Part print with two shaded views. Sizes in mm from the minimum x, y, z corner. A direction names the side the tool comes from. Give positions to 0.01 mm unless a question says otherwise; leave off trailing zeros. Order: outer loops, then holes, each group sorted by start corner. A loop starts at its lowest first (then second) coordinate and runs counter-clockwise, first axis right, second up. Notation, with made-up numbers: (-39, 4.5) -> (-2, 4.5) arc R17 ccw to (-2, 9.5) -> close; hole circle Ø3 at (37, 44.5). An arc over 180 degrees is marked (long way). Write item = value, one per line. Start each with the question number.
Item 1: Drill centre lines: line 1 along Z through (x, y) = (4.5, 25); line 2 along X through (y, z) = (29, 10.5); line 3 along Y through (x, z) = (79.5, 38.5). Where is each one in solid material? Low to high.
Item 2: Band-saw the part on B-B on z = 32.5. Write the cut outline in (x, y), plus the area to 3 significant figures.
Item 3: Band-saw the part on A-A on y = 7. Write the cut outline in (x, z).
Item 4: Flat gauge pins, fed straight in: P1, Ø15, axis at x = 75.5, z = 42, coming from the +Y side; P2, Ø3, axis at x = 14, y = 53, coming from the +Z side; P3, Ø6, axis at y = 11.5, z = 34.5, coming from the +X side. Where does each tip first touch, or does it go through?
Item 5: Band-saw the part on D-D on y = 43. Write the cut outline in (x, z), plus the area to 3 significant figures.
Item 6: Tool access for the marked faces 1, 2 and 3: list every direction of +Z, -Z, +X, -X, +Y, -Y with a clear straight run to the whole face (end or side of a thin tool).
Item 7: Band-saw the part on C-C on x = 62. Write the cut outline in (y, z), plus the area to 3 significant figures.
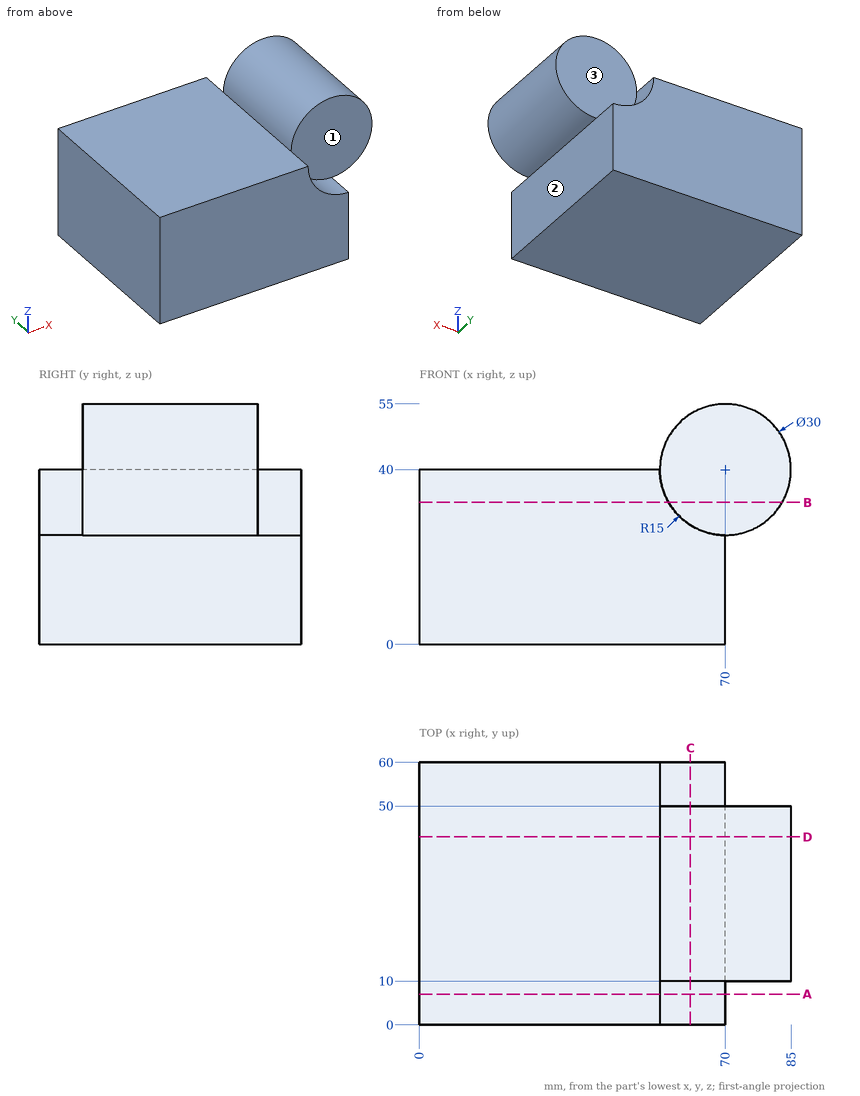
Values found:
q1.line_1 = 0 to 40
q1.line_2 = 0 to 70
q1.line_3 = 10 to 50
q2.outline = (0, 0) -> (57.01, 0) -> (57.01, 10) -> (82.99, 10) -> (82.99, 50) -> (57.01, 50) -> (57.01, 60) -> (0, 60) -> close
q2.area = 4,460 mm^2
q3.outline = (0, 0) -> (70, 0) -> (70, 25) arc R15 cw to (55, 40) -> (0, 40) -> close
q4.P1 = 50
q4.P2 = 40
q4.P3 = 84.79
q5.outline = (0, 0) -> (70, 0) -> (70, 25) arc R15 ccw (long way) to (55, 40) -> (0, 40) -> close
q5.area = 3,330 mm^2
q6.face_1 = +Z, +X, -Y
q6.face_2 = -Z, +X, +Y, -Y
q6.face_3 = +Z, +X, +Y
q7.outline = (0, 0) -> (60, 0) -> (60, 27.31) -> (50, 27.31) -> (50, 52.69) -> (10, 52.69) -> (10, 27.31) -> (0, 27.31) -> close
q7.area = 2,650 mm^2
